CAD build for the part. Positions are in the model's coordinates, mm. A direction names the side the tool comes from. Coordinates: 2 decimals unless noted, no trailing zeros. Order: outer loops, then holes, each group sorted by start corner. A loop starts at its lowest first (then second) coordinate and runs counter-clockwise, first axis right, second up. Notation, with made-up numbers: M 44,5.5 L 97,5.5 A26 ccw 97,39.5 Z; hole C 51.5,48.5 d7. An arc over 180 degrees is marked long. Write item = value, one per line.
from build123d import *

# Parameters (mm, degrees)
BOSS_EXTRU_1_DEPTH      = 3
ESQUISSE2_W             = 20
ESQUISSE2_H             = 3
BOSS_EXTRU_2_DEPTH      = 32
ESQUISSE3_R             = 0.6
ENL_V_MAT_EXTRU_1_DEPTH = 32


with BuildPart() as part:
    # Esquisse1 → Boss.-Extru.1 (new body)
    with BuildSketch(Plane(origin=(0, 0, 0), x_dir=(1, 0, 0), z_dir=(0, 1, 0))):
        with BuildLine():
            Line((-1.600915354, 17.472527473), (-21.600915354, 17.472527473))
            Line((-21.600915354, 17.472527473), (-21.600915354, -22.527472527))
            Line((-21.600915354, -22.527472527), (-1.600915354, -22.527472527))
            Line((-1.600915354, -22.527472527), (-1.600915354, -14.527472527))
            ThreePointArc((-1.600915354, -14.527472527), (-10.086196728, -11.012753902), (-13.600915354, -2.527472527))
            ThreePointArc((-13.600915354, -2.527472527), (-10.086196728, 5.957808847), (-1.600915354, 9.472527473))
            Line((-1.600915354, 9.472527473), (-1.600915354, 17.472527473))
        make_face()
        with BuildLine():
            Line((-12.100915354, -2.527472527), (-13.600915354, -2.527472527))
            ThreePointArc((-13.600915354, -2.527472527), (-10.086196728, -11.012753902), (-1.600915354, -14.527472527))
            Line((-1.600915354, -14.527472527), (-1.600915354, -13.627472527))
            ThreePointArc((-1.600915354, -13.627472527), (-2.031197653, -13.445631759), (-2.200670406, -13.01032967))
            ThreePointArc((-2.200670406, -13.01032967), (-3.255915354, -12.896222452), (-4.294249093, -12.676164727))
            ThreePointArc((-4.294249093, -12.676164727), (-5.0563189, -13.075940963), (-5.434158505, -12.302760091))
            ThreePointArc((-5.434158505, -12.302760091), (-10.275563851, -8.443592325), (-12.100915354, -2.527472527))
        make_face()
        with BuildLine():
            Line((-1.600915354, 8.572527473), (-1.600915354, 9.472527473))
            ThreePointArc((-1.600915354, 9.472527473), (-10.086196728, 5.957808847), (-13.600915354, -2.527472527))
            Line((-13.600915354, -2.527472527), (-12.100915354, -2.527472527))
            ThreePointArc((-12.100915354, -2.527472527), (-10.275563851, 3.38864727), (-5.434158505, 7.247815036))
            ThreePointArc((-5.434158505, 7.247815036), (-5.0563189, 8.020995908), (-4.294249093, 7.621219672))
            ThreePointArc((-4.294249093, 7.621219672), (-3.255915354, 7.841277397), (-2.200670406, 7.955384615))
            ThreePointArc((-2.200670406, 7.955384615), (-2.031197653, 8.390686704), (-1.600915354, 8.572527473))
        make_face()
        with BuildLine():
            Line((-11.700915354, -2.527472527), (-12.100915354, -2.527472527))
            ThreePointArc((-12.100915354, -2.527472527), (-10.275563851, -8.443592325), (-5.434158505, -12.302760091))
            ThreePointArc((-5.434158505, -12.302760091), (-4.766513404, -11.914665117), (-4.26954033, -12.50575348))
            ThreePointArc((-4.26954033, -12.50575348), (-4.27141827, -12.553187658), (-4.277040334, -12.600324908))
            Line((-4.277040334, -12.600324908), (-2.193415349, -12.932901099))
            ThreePointArc((-2.193415349, -12.932901099), (-1.990310489, -12.570995334), (-1.600915354, -12.427472527))
            Line((-1.600915354, -12.427472527), (-1.600915354, -12.027472527))
            ThreePointArc((-1.600915354, -12.027472527), (-6.796887474, -10.480577187), (-10.300728002, -6.34365647))
            ThreePointArc((-10.300728002, -6.34365647), (-11.087859343, -5.99271332), (-10.712234442, -5.217056968))
            ThreePointArc((-10.712234442, -5.217056968), (-10.955645441, -4.182472527), (-11.081967985, -3.127173284))
            ThreePointArc((-11.081967985, -3.127173284), (-11.518426778, -2.958383435), (-11.700915354, -2.527472527))
        make_face()
        with BuildLine():
            ThreePointArc((-5.434158505, 7.247815036), (-10.275563851, 3.38864727), (-12.100915354, -2.527472527))
            Line((-12.100915354, -2.527472527), (-11.700915354, -2.527472527))
            ThreePointArc((-11.700915354, -2.527472527), (-11.518426778, -2.09656162), (-11.081967985, -1.927771771))
            ThreePointArc((-11.081967985, -1.927771771), (-10.955645441, -0.872472527), (-10.712234442, 0.162111913))
            ThreePointArc((-10.712234442, 0.162111913), (-11.087859343, 0.937768265), (-10.300728002, 1.288711415))
            ThreePointArc((-10.300728002, 1.288711415), (-6.796887474, 5.425632132), (-1.600915354, 6.972527473))
            Line((-1.600915354, 6.972527473), (-1.600915354, 7.372527473))
            ThreePointArc((-1.600915354, 7.372527473), (-1.990310489, 7.516050279), (-2.193415349, 7.877956044))
            Line((-2.193415349, 7.877956044), (-4.277040334, 7.545379853))
            ThreePointArc((-4.277040334, 7.545379853), (-4.27141827, 7.498242603), (-4.26954033, 7.450808425))
            ThreePointArc((-4.26954033, 7.450808425), (-4.766513404, 6.859720062), (-5.434158505, 7.247815036))
        make_face()
        with BuildLine():
            Line((-1.600915354, -2.527472527), (-1.600915354, 6.972527473))
            ThreePointArc((-1.600915354, 6.972527473), (-6.796887474, 5.425632132), (-10.300728002, 1.288711415))
            ThreePointArc((-10.300728002, 1.288711415), (-10.027222023, 1.06797018), (-9.924278512, 0.731912377))
            ThreePointArc((-9.924278512, 0.731912377), (-10.138737197, 0.27217561), (-10.628804827, 0.141087318))
            Line((-10.628804827, 0.141087318), (-10.996389038, -1.936647469))
            ThreePointArc((-10.996389038, -1.936647469), (-10.641178587, -2.141931213), (-10.500915354, -2.527472527))
            ThreePointArc((-10.500915354, -2.527472527), (-10.641178587, -2.913013842), (-10.996389038, -3.118297586))
            Line((-10.996389038, -3.118297586), (-10.628804827, -5.196032373))
            ThreePointArc((-10.628804827, -5.196032373), (-10.138737197, -5.327120665), (-9.924278512, -5.786857431))
            ThreePointArc((-9.924278512, -5.786857431), (-10.027222023, -6.122915235), (-10.300728002, -6.34365647))
            ThreePointArc((-10.300728002, -6.34365647), (-6.796887474, -10.480577187), (-1.600915354, -12.027472527))
            Line((-1.600915354, -12.027472527), (-1.600915354, -2.527472527))
        make_face()
        with BuildLine():
            ThreePointArc((7.098897295, 1.288711415), (3.595056766, 5.425632132), (-1.600915354, 6.972527473))
            Line((-1.600915354, 6.972527473), (-1.600915354, -2.527472527))
            Line((-1.600915354, -2.527472527), (-1.600915354, -12.027472527))
            ThreePointArc((-1.600915354, -12.027472527), (3.595056766, -10.480577187), (7.098897295, -6.34365647))
            ThreePointArc((7.098897295, -6.34365647), (6.745557904, -5.621939139), (7.42697412, -5.196032373))
            Line((7.42697412, -5.196032373), (7.794558331, -3.118297586))
            ThreePointArc((7.794558331, -3.118297586), (7.299084646, -2.527472527), (7.794558331, -1.936647469))
            Line((7.794558331, -1.936647469), (7.42697412, 0.141087318))
            ThreePointArc((7.42697412, 0.141087318), (6.745557904, 0.566994084), (7.098897295, 1.288711415))
        make_face()
        with BuildLine():
            ThreePointArc((2.232327798, -12.302760091), (7.073733143, -8.443592325), (8.899084646, -2.527472527))
            Line((8.899084646, -2.527472527), (8.499084646, -2.527472527))
            ThreePointArc((8.499084646, -2.527472527), (8.316596071, -2.958383435), (7.880137278, -3.127173284))
            ThreePointArc((7.880137278, -3.127173284), (7.753814733, -4.182472527), (7.510403735, -5.217056968))
            ThreePointArc((7.510403735, -5.217056968), (7.80864404, -5.435270713), (7.922447804, -5.786857431))
            ThreePointArc((7.922447804, -5.786857431), (7.658505607, -6.28391392), (7.098897295, -6.34365647))
            ThreePointArc((7.098897295, -6.34365647), (3.595056766, -10.480577187), (-1.600915354, -12.027472527))
            Line((-1.600915354, -12.027472527), (-1.600915354, -12.427472527))
            ThreePointArc((-1.600915354, -12.427472527), (-1.211520218, -12.570995334), (-1.008415358, -12.932901099))
            Line((-1.008415358, -12.932901099), (1.075209627, -12.600324908))
            ThreePointArc((1.075209627, -12.600324908), (1.518275509, -11.92466016), (2.232327798, -12.302760091))
        make_face()
        with BuildLine():
            Line((8.499084646, -2.527472527), (8.899084646, -2.527472527))
            ThreePointArc((8.899084646, -2.527472527), (7.073733143, 3.38864727), (2.232327798, 7.247815036))
            ThreePointArc((2.232327798, 7.247815036), (1.518275509, 6.869715106), (1.075209627, 7.545379853))
            Line((1.075209627, 7.545379853), (-1.008415358, 7.877956044))
            ThreePointArc((-1.008415358, 7.877956044), (-1.211520218, 7.516050279), (-1.600915354, 7.372527473))
            Line((-1.600915354, 7.372527473), (-1.600915354, 6.972527473))
            ThreePointArc((-1.600915354, 6.972527473), (3.595056766, 5.425632132), (7.098897295, 1.288711415))
            ThreePointArc((7.098897295, 1.288711415), (7.658505607, 1.228968865), (7.922447804, 0.731912377))
            ThreePointArc((7.922447804, 0.731912377), (7.80864404, 0.380325658), (7.510403735, 0.162111913))
            ThreePointArc((7.510403735, 0.162111913), (7.753814733, -0.872472527), (7.880137278, -1.927771771))
            ThreePointArc((7.880137278, -1.927771771), (8.316596071, -2.09656162), (8.499084646, -2.527472527))
        make_face()
        with BuildLine():
            ThreePointArc((10.399084646, -2.527472527), (6.884366021, 5.957808847), (-1.600915354, 9.472527473))
            Line((-1.600915354, 9.472527473), (-1.600915354, 8.572527473))
            ThreePointArc((-1.600915354, 8.572527473), (-1.176651285, 8.396791541), (-1.000915354, 7.972527473))
            ThreePointArc((-1.000915354, 7.972527473), (-1.000976594, 7.963955169), (-1.001160302, 7.955384615))
            ThreePointArc((-1.001160302, 7.955384615), (0.054084646, 7.841277397), (1.092418386, 7.621219672))
            ThreePointArc((1.092418386, 7.621219672), (1.753806249, 8.044599104), (2.267709623, 7.450808425))
            ThreePointArc((2.267709623, 7.450808425), (2.258797985, 7.347781499), (2.232327798, 7.247815036))
            ThreePointArc((2.232327798, 7.247815036), (7.073733143, 3.38864727), (8.899084646, -2.527472527))
            Line((8.899084646, -2.527472527), (10.399084646, -2.527472527))
        make_face()
        with BuildLine():
            ThreePointArc((-1.600915354, -14.527472527), (6.884366021, -11.012753902), (10.399084646, -2.527472527))
            Line((10.399084646, -2.527472527), (8.899084646, -2.527472527))
            ThreePointArc((8.899084646, -2.527472527), (7.073733143, -8.443592325), (2.232327798, -12.302760091))
            ThreePointArc((2.232327798, -12.302760091), (2.258797985, -12.402726554), (2.267709623, -12.50575348))
            ThreePointArc((2.267709623, -12.50575348), (1.753806249, -13.099544159), (1.092418386, -12.676164727))
            ThreePointArc((1.092418386, -12.676164727), (0.054084646, -12.896222452), (-1.001160302, -13.01032967))
            ThreePointArc((-1.001160302, -13.01032967), (-1.000976594, -13.018900224), (-1.000915354, -13.027472527))
            ThreePointArc((-1.000915354, -13.027472527), (-1.176651285, -13.451736596), (-1.600915354, -13.627472527))
            Line((-1.600915354, -13.627472527), (-1.600915354, -14.527472527))
        make_face()
        with BuildLine():
            Line((18.399084646, 17.472527473), (-1.600915354, 17.472527473))
            Line((-1.600915354, 17.472527473), (-1.600915354, 9.472527473))
            ThreePointArc((-1.600915354, 9.472527473), (6.884366021, 5.957808847), (10.399084646, -2.527472527))
            ThreePointArc((10.399084646, -2.527472527), (6.884366021, -11.012753902), (-1.600915354, -14.527472527))
            Line((-1.600915354, -14.527472527), (-1.600915354, -22.527472527))
            Line((-1.600915354, -22.527472527), (18.399084646, -22.527472527))
            Line((18.399084646, -22.527472527), (18.399084646, 17.472527473))
        make_face()
    extrude(amount=BOSS_EXTRU_1_DEPTH)

    # Esquisse2 → Boss.-Extru.2 (add)
    with BuildSketch(Plane(origin=(0, 3, 0), x_dir=(1, 0, 0), z_dir=(0, 1, 0))):
        with Locations((-11.600915354, 15.972527473)):
            Rectangle(ESQUISSE2_W, ESQUISSE2_H)
        with Locations((8.399084646, 15.972527473)):
            Rectangle(ESQUISSE2_W, ESQUISSE2_H)
    extrude(amount=BOSS_EXTRU_2_DEPTH)

    # Esquisse3 → Enlèv. mat.-Extru.1 (cut)
    with BuildSketch(Plane.XY.offset(-14.472527473)):
        with Locations((7.362779374, 22.8773094)):
            Circle(ESQUISSE3_R)
        with Locations((-11.637220626, 22.8773094)):
            Circle(ESQUISSE3_R)
        with Locations((-2.137220626, 33.3773094)):
            Circle(ESQUISSE3_R)
        with Locations((-2.137220626, 12.3773094)):
            Circle(ESQUISSE3_R)
        with Locations((1.13140435, 32.855590352)):
            Circle(ESQUISSE3_R)
        with Locations((-5.405845603, 32.855590352)):
            Circle(ESQUISSE3_R)
        with Locations((-5.405845603, 12.899028447)):
            Circle(ESQUISSE3_R)
        with Locations((1.13140435, 12.899028447)):
            Circle(ESQUISSE3_R)
        with Locations((-11.060583784, 26.136694304)):
            Circle(ESQUISSE3_R)
        with Locations((-11.060583784, 19.617924496)):
            Circle(ESQUISSE3_R)
        with Locations((6.786142531, 26.136694304)):
            Circle(ESQUISSE3_R)
        with Locations((6.786142531, 19.617924496)):
            Circle(ESQUISSE3_R)
    extrude(amount=-ENL_V_MAT_EXTRU_1_DEPTH, mode=Mode.SUBTRACT)


solid = part.part
(1) Slice it at A-A, the plane x = -3.5. Write the cut outline in (y, z), then the cut area to 3 significant figures.
Evaluation:
outline = M 0,-17.47 L 35,-17.47 L 35,-14.47 L 3,-14.47 L 3,-7.8 L 0,-7.8 Z; M 0,-7.67 L 3,-7.67 L 3,12.72 L 0,12.72 Z; M 0,12.85 L 3,12.85 L 3,22.53 L 0,22.53 Z
area = 215 mm²
(2) Pull direction X, two halves, no side cores. Call faces 1 (the face through (-2, 1, 22.527)), 2 (the face through (-2.22, 12.97, -15.95)), 3 (the face through (1.001, 12.313, -15.952)), 4 (the face through (18.399, 2, -6)): +X half, -X half, draft (parallel to the pull), parting line (faces both ways), or undercut.
Evaluation:
face_1 = draft
face_2 = undercut
face_3 = undercut
face_4 = +X half
(3) Tool access for faces 5 (the face through (7.3, 1.5, 2.5)), 6 (the face through (-2, 0, 2)): list every direction of +Z, -Z, +X, -X, +Y, -Y with a clear straight run to the whole face (end or side of a thin tool).
Evaluation:
face_5 = +Y, -Y
face_6 = +Z, -Z, +X, -X, -Y
(4) Slice it at B-B, the plane x = -18. Write the cut outline in (y, z).
Evaluation:
outline = M 0,-17.47 L 35,-17.47 L 35,-14.47 L 3,-14.47 L 3,22.53 L 0,22.53 Z
(5) Slice it at C-C, the plane z = 18.5. Write the cut outline in (x, y), then the cut area to 3 significant figures.
Evaluation:
outline = M -21.6,0 L 18.4,0 L 18.4,3 L -21.6,3 Z
area = 120 mm²
(6) Wall check: line 1 (Y direction, x = 15, z = -7); line 2 (Z direction, x = -4, y = 19). Give the ranges that are in metal, low to high. Write a range as from..to.
Evaluation:
line_1 = 0..3
line_2 = -17.47..-14.47
(7) Pin check, flat tips, straight feed: pin 1 Ø1.4 at (x, y) = (6.79, 19.62) entering from +Z; pin 2 Ø1.1 at (x, y) = (6.79, 26.14) entering from +Z; pin 3 Ø6 at (x, z) = (-14.5, 5) entering from +Y. Stop position of each tip, or through.
Evaluation:
pin_1 = -14.47
pin_2 = through
pin_3 = 3
(8) Slice it at D-D, the plane y = 5.5. Write the cut outline in (x, z).
Evaluation:
outline = M -21.6,-17.47 L 18.4,-17.47 L 18.4,-14.47 L -21.6,-14.47 Z
